```python
from build123d import *

# Parameters (mm, degrees)
SKETCH1_R                = 20.675
SKETCH1_R_2              = 17.5
SKETCH3_R                = 2.5
CUT_EXTRUDE1_DEPTH       = 21.675
CUT_EXTRUDE1_DEPTH_BACK  = 21.675
BOSS_EXTRUDE1_DEPTH      = 7.5
BOSS_EXTRUDE1_DEPTH_BACK = 7.5
SKETCH5_R                = 5
CUT_EXTRUDE2_DEPTH       = 10.1750001
CUT_EXTRUDE2_DEPTH_BACK  = 33.1750001


with BuildPart() as part:
    # Sweep1: sweep along a path in Sketch2
    with BuildLine(Plane(origin=(0, 0, 0), x_dir=(0, 0, -1), z_dir=(1, 0, 0))) as sweep1_path:
        Line((0, 0), (-50, 0))
        Line((-50, 0), (-98.168231432, 40.417945229))
    # Sketch1 → Sweep1 (sweep)
    with BuildSketch(Plane.XY):
        Circle(SKETCH1_R)
        Circle(SKETCH1_R_2, mode=Mode.SUBTRACT)
    sweep(path=sweep1_path.line, transition=Transition.RIGHT)

    # Sketch3 → Cut-Extrude1 (cut, two sides)
    with BuildSketch(Plane(origin=(0, 0, 0), x_dir=(0, 0, -1), z_dir=(1, 0, 0))) as cut_extrude1_sk:
        with Locations((-86.677564785, 30.776131084)):
            Circle(SKETCH3_R)
        with Locations((-15, 0)):
            Circle(SKETCH3_R)
    extrude(amount=CUT_EXTRUDE1_DEPTH, mode=Mode.SUBTRACT)
    extrude(cut_extrude1_sk.sketch, amount=-CUT_EXTRUDE1_DEPTH_BACK, mode=Mode.SUBTRACT)

    # Sketch4 → Boss-Extrude1 (add, two sides)
    with BuildSketch(Plane(origin=(0, 0, 15), x_dir=(-1, 0, 0), z_dir=(0, 0, -1))) as boss_extrude1_sk:
        with BuildLine():
            Line((-11.5, 39.18154897), (-7.5, 39.18154897))
            Line((-7.5, 39.18154897), (-7.5, 24.18154897))
            ThreePointArc((-7.5, 24.18154897), (-7.207106781, 23.474442189), (-6.5, 23.18154897))
            Line((-6.5, 23.18154897), (6.5, 23.18154897))
            ThreePointArc((6.5, 23.18154897), (7.207106781, 23.474442189), (7.5, 24.18154897))
            Line((7.5, 24.18154897), (7.5, 39.18154897))
            Line((7.5, 39.18154897), (11.5, 39.18154897))
            Line((11.5, 39.18154897), (11.5, 17.18154897))
            Line((11.5, 17.18154897), (8.31426673, 17.18154897))
            ThreePointArc((8.31426673, 17.18154897), (0, 19.0875), (-8.31426673, 17.18154897))
            Line((-8.31426673, 17.18154897), (-11.5, 17.18154897))
            Line((-11.5, 17.18154897), (-11.5, 39.18154897))
        make_face()
    extrude(amount=BOSS_EXTRUDE1_DEPTH)
    extrude(boss_extrude1_sk.sketch, amount=-BOSS_EXTRUDE1_DEPTH_BACK)

    # Sketch5 → Cut-Extrude2 (cut, two sides)
    with BuildSketch(Plane(origin=(11.5, 0, 0), x_dir=(0, 0, -1), z_dir=(1, 0, 0))) as cut_extrude2_sk:
        with Locations((-15, 31.68154897)):
            Circle(SKETCH5_R)
    extrude(amount=CUT_EXTRUDE2_DEPTH, mode=Mode.SUBTRACT)
    extrude(cut_extrude2_sk.sketch, amount=-CUT_EXTRUDE2_DEPTH_BACK, mode=Mode.SUBTRACT)


solid = part.part
```
Can you work these out from the model? Positions are in its coordinate system, mm. A direction names the side the tool comes from. Coordinates: 2 decimals unless noted, no trailing zeros. Loops run counter-clockwise (first coordinate to the right, second up) from the corner with the lowest first, then second, coordinate; pieces in that order, holes last.
1) Imagine slicing it at A-A on x = 14.5. List the corners of the cut face in (y, z) for me.
2) Which directions (+Z, -Z, +X, -X, +Y, -Y) give clear straight access to the entire face, cutting with the end or side of a thin tool? Please do faces 1 (the flat face through (-17, 5, 0)), 2 (the flat face through (-9, 39.182, 15)), 3 (the cylindrical face through (-18.97, -2.44, 15.54)), 4 (the flat face through (7.5, 37, 15)), 5 (the cylindrical face through (8.075, -15.526, 28.579)).
3) Thinking about a two-plate mould opening in X: for faces 6 (the flat face through (-11.5, 26, 15)), 7 (the cylindrical face through (9.53, 26.8, 16.08)), 8 (the flat face through (0, 23.182, 15)), 9 (the cylindrical face through (-4.482, -20.183, 29.165)), which applies, pulls with the +X half, pulls with the -X half, needs draft (parallel to the pull), parting line crosses it, or undercut?
4) For pin 1 (12 mm diameter, centred on y = 29, z = 11.5, fed in from +X); pin 2 (5 mm diameter, centred on x = 3, z = 17, fed in from +Y); pin 3 (4 mm diameter, centred on x = 9, y = -3, fed in from +Z), each with a flat end and sliding along its axis, tell me the tip position at first contact or that it passes through.
5) Imagine slicing it at C-C on z = 34.5. List the corners of the cut face in (x, y) for me (3 decimals).
6) Imagine slicing it at D-D on x = -4. List the corners of the cut face in (y, z) for me.
7) I need wall thicknesses on probe 1 along Y at (x, z) = (-9.1, 15); probe 2 along X at (y, z) = (15, 68.5); probe 3 along Y at (x, z) = (0, 12) (3 decimals). Which ranges of each line are inside material? Lowest first, please.
8) Imagine slicing it at B-B on z = 15. State how many separate pieces and enclosed holes the cut face has, plus the area to 3 significant figures.
Completed:
1. outline: (-14.74, 0) - (-9.8, 0) - (-9.8, 53.57) - (32.91, 104.47) - (29.13, 107.64) - (-14.74, 55.36) - close; (9.8, 0) - (14.74, 0) - (14.74, 44.64) - (51.71, 88.69) - (47.92, 91.87) - (9.8, 46.43) - close
2. face 1: -Z, +X, -X, +Y, -Y
2. face 2: -Z, +X, -X, +Y
2. face 3: +X, -X
2. face 4: -Z, +Y
2. face 5: -Z
3. face 6: pulls with the -X half
3. face 7: needs draft
3. face 8: undercut
3. face 9: parting line crosses it
4. pin 1: stops at x = 11.5
4. pin 2: stops at y = 23.18
4. pin 3: stops at z = 78.15
5. outline: circle Ø41.35 at (0, 0); hole circle Ø35 at (0, 0)
6. outline: (-20.28, 0) - (-17.04, 0) - (-17.04, 56.2) - (27.37, 109.12) - (24.88, 111.21) - (-20.28, 57.38) - close; (17.04, 0) - (20.28, 0) - (20.28, 7.5) - (23.18, 7.5) - (23.18, 22.5) - (20.28, 22.5) - (20.28, 42.62) - (55.96, 85.13) - (53.47, 87.22) - (17.04, 43.8) - close
7. probe 1: y = -18.56 to -14.95, 14.95 to 26.68, 36.68 to 39.18
7. probe 2: x = -20.67 to -17.5, 17.5 to 20.67
7. probe 3: y = -20.675 to -17.5, 17.5 to 23.182
8. separate pieces: 4
8. enclosed holes: 0
8. area: 481 mm2
